Input: dimensioned drawing with shaded views. Units: mm. Origin: part minimum x, y, z. Round coordinates to 2 decimals unless told otherwise and drop trailing zeros. Loops run counter-clockwise (first coordinate to the right, second up) from the corner with the lowest first, then second, coordinate; pieces in that order, holes last. Notation, with made-up numbers: M -35,-15 L 11,-15 A19 ccw 11,8 Z; hole C 23,-33.5 d7. An arc over 180 degrees is marked long. Return JSON: item names as keys, results as strings.
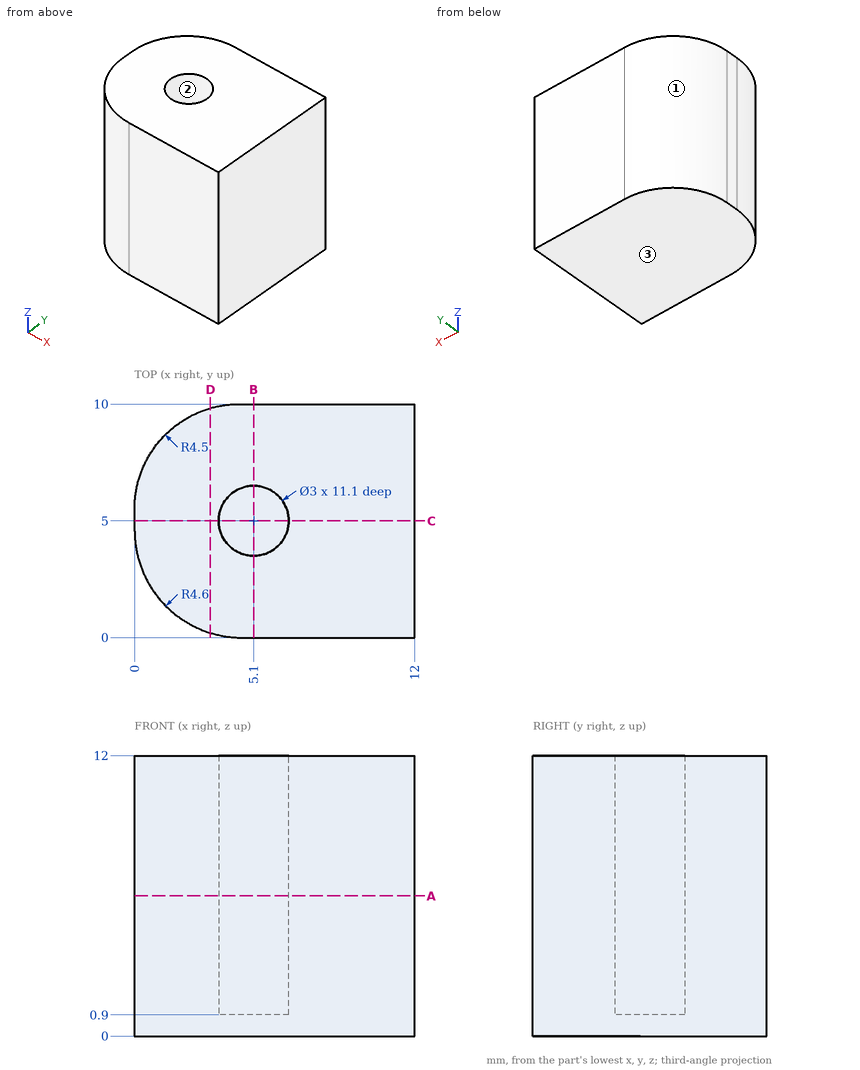
Q1. Section query C-C (y = 5). Output: boundary loops of the cut face in (x, z), plus the area to 3 significant figures.
Determined:
{"outline": "M 0,0 L 12,0 L 12,12 L 6.6,12 L 6.6,0.9 L 3.6,0.9 L 3.6,12 L 0,12 Z", "area": "111 mm^2"}
Q2. Pin query (flat end, axial travel): pin 1 (2.5 mm diameter, centred on x = 5.1, y = 5, fed in from -Z); pin 2 (1 mm diameter, centred on y = 8.5, z = 10.5, fed in from -X). Return the tip coordinate at first contact, or that it passes through.
Determined:
{"pin 1": "stops at z = 0", "pin 2": "stops at x = 0.76"}
Q3. Section query D-D (x = 3.25). Output: boundary loops of the cut face in (y, z), plus the area to 3 significant figures.
Determined:
{"outline": "M 0.2,0 L 9.82,0 L 9.82,12 L 0.2,12 Z", "area": "115 mm^2"}
Q4. Section query B-B (x = 5.1). Output: boundary loops of the cut face in (y, z).
Determined:
{"outline": "M 0,0 L 10,0 L 10,12 L 6.5,12 L 6.5,0.9 L 3.5,0.9 L 3.5,12 L 0,12 Z"}
Q5. Material intervals for L1, parallel to Y at x = 5.1, z = 3.5; L2, parallel to X at y = 5, z = 8.5; L3, parallel to Z at x = 4.5, y = 6.25, sorted ascending.
Determined:
{"L1": "y = 0 to 3.5, 6.5 to 10", "L2": "x = 0 to 3.6, 6.6 to 12", "L3": "z = 0 to 0.9"}
Q6. Section query A-A (z = 6). Output: boundary loops of the cut face in (x, y).
Determined:
{"outline": "M 0,4.6 A4.6 ccw 4.6,0 L 12,0 L 12,10 L 4.5,10 A4.5 ccw 0,5.5 Z; hole C 5.1,5 d3"}
Q7. Pull-direction query (X, two-part tool) for the marked faces 1, 2 and 3; classes: pulls with the +X half, pulls with the -X half, needs draft (parallel to the pull), parting line crosses it, or undercut.
Determined:
{"face 1": "pulls with the -X half", "face 2": "undercut", "face 3": "needs draft"}
